Answer from the drawing. Dimensions are ordinates in mm from the lowest x, y and z of the part. A direction names the side the tool comes from. Coordinates: 2 decimals unless noted, no trailing zeros. Order: outer loops, then holes, each group sorted by start corner. A loop starts at its lowest first (then second) coordinate and runs counter-clockwise, first axis right, second up. Notation, with made-up numbers: (3.5, 47.25) -> (60.5, 47.25) arc R20 ccw to (60.5, 68.25) -> close; hole circle Ø5 at (26, 13). An arc over 180 degrees is marked (long way). Answer in a Markdown table with one row per item.
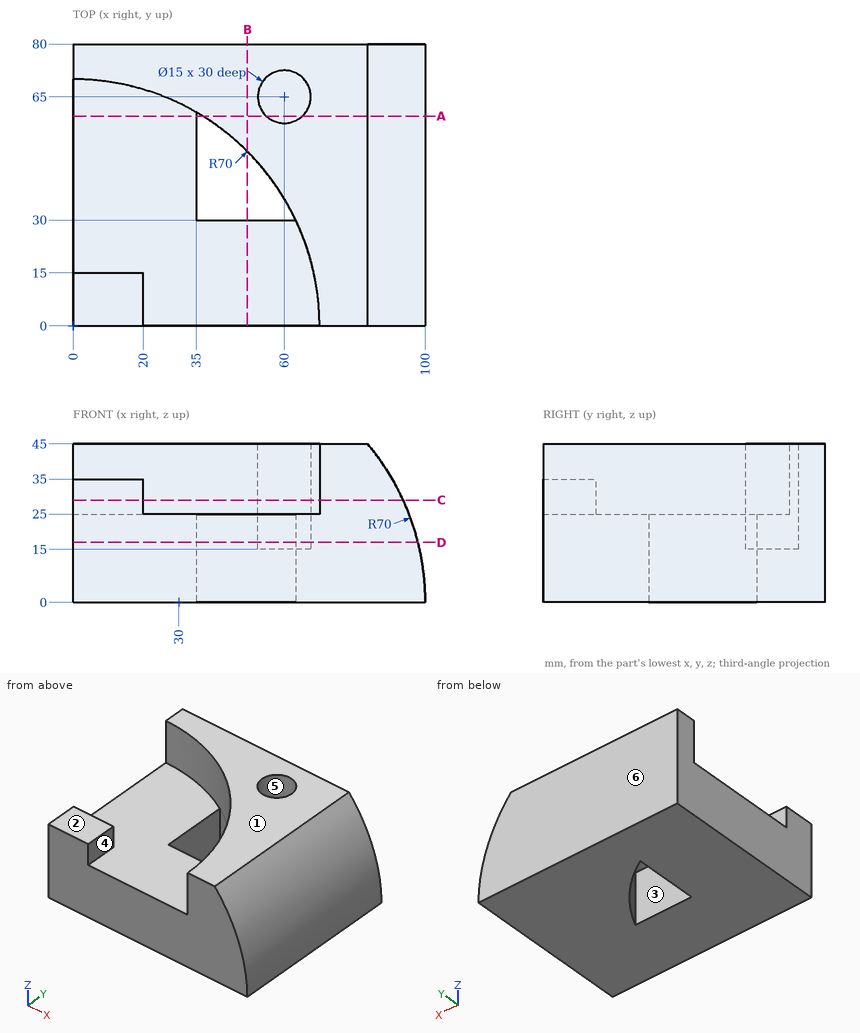
(1) A cutting plane is placed at C-C, the plane z = 29. Determine the outline of the cut face in (x, y).
Check values:
| item | result |
|---|---|
| outline | (0, 0) -> (20, 0) -> (20, 15) -> (0, 15) -> close; (0, 70) arc R70 cw to (70, 0) -> (93.71, 0) -> (93.71, 80) -> (0, 80) -> close; hole circle Ø15 at (60, 65) |
(2) A cutting plane is placed at A-A, the plane y = 59.5. Determine the outline of the cut face in (x, z), then the cut area to 3 significant figures.
Check values:
| item | result |
|---|---|
| outline | (0, 0) -> (35, 0) -> (35, 25) -> (0, 25) -> close; (36.87, 0) -> (100, 0) arc R70 ccw to (83.62, 45) -> (65.1, 45) -> (65.1, 15) -> (54.9, 15) -> (54.9, 45) -> (36.87, 45) -> close |
| area | 3,180 mm² |
(3) For a pull along Y with two mould halves and no side action, classify the marked faces 4, 5 and 6 as released by +Y, released by -Y, zero draft, split by the parting line, or undercut.
Check values:
| item | result |
|---|---|
| face 4 | zero draft |
| face 5 | undercut |
| face 6 | released by +Y |
(4) Flat-ended cylindrical pins translate along their axes: pin 1 (10 mm diameter, centred on y = 51, z = 22.5, fed in from +X); pin 2 (3 mm diameter, centred on y = 6, z = 30.5, fed in from +X); pin 3 (16.5 mm diameter, centred on x = 10.5, y = 5, fed in from +Z). Find the tip coordinate at first contact, or state that the pin passes through.
Check values:
| item | result |
|---|---|
| pin 1 | x = 97.78 |
| pin 2 | x = 93.71 |
| pin 3 | z = 35 |
(5) Which of the six approach directions +Z, -Z, +X, -X, +Y, -Y give full straight-line access (tool end or side, diameter ignored) to the marked faces 1, 2 and 3?
Check values:
| item | result |
|---|---|
| face 1 | +Z, +X, -X, +Y, -Y |
| face 2 | +Z, -X, -Y |
| face 3 | +Z, -Z |
(6) Find the intervals of material crossed by line 1 along Z through (x, y) = (35, 17); line 2 along Y through (x, z) = (39.5, 9); line 3 along Y through (x, z) = (60, 34.25), in increasing order. Write a range as from..to.
Check values:
| item | result |
|---|---|
| line 1 | 0..25 |
| line 2 | 0..30, 57.79..80 |
| line 3 | 36.06..57.5, 72.5..80 |
(7) A cutting plane is placed at D-D, the plane z = 17. Determine the outline of the cut face in (x, y), then the cut area to 3 significant figures.
Check values:
| item | result |
|---|---|
| outline | (0, 0) -> (97.9, 0) -> (97.9, 80) -> (0, 80) -> close; hole (35, 30) -> (63.25, 30) arc R70 ccw to (35, 60.62) -> close; hole circle Ø15 at (60, 65) |
| area | 7,130 mm² |
(8) A cutting plane is placed at B-B, the plane x = 49.5. Determine the outline of the cut face in (y, z), then the cut area to 3 significant figures.
Check values:
| item | result |
|---|---|
| outline | (0, 0) -> (30, 0) -> (30, 25) -> (0, 25) -> close; (49.49, 0) -> (80, 0) -> (80, 45) -> (49.49, 45) -> close |
| area | 2,120 mm² |
